Could you check a few things on this model? Use its own coordinates, in mm. A direction names the side the tool comes from. Give positions to 0.01 mm unless a question says otherwise; leave off trailing zeros. Order: outer loops, then holes, each group sorted by start corner. A loop starts at its lowest first (then second) coordinate and runs counter-clockwise, first axis right, second up.
from build123d import *

# Parameters (mm, degrees)
ENL_V_MAT_EXTRU_1_DEPTH = 0.5
CONG_1_R                = 0.2
CONG_2_R                = 1


# Read off the part's stored shape, not the designer's step: M5 Filetages mécaniques Borne1
with BuildPart() as part:
    # Esquisse1 → Révolution1 (revolve)
    with BuildSketch(Plane.XY):
        with BuildLine():
            Line((0, 0), (-7, 0))
            ThreePointArc((-7, 0), (-6.746211251, 2.061552813), (-6, 4))
            Line((-6, 4), (-5, 4))
            Line((-5, 4), (-5, 3))
            Line((-5, 3), (0, 3))
            Line((0, 3), (0, 0))
        make_face()
    revolve(axis=Axis((0, 0, 0), (-1, 0, 0)))

    # Esquisse2 → Enlèv. mat.-Extru.1 (cut)
    with BuildSketch(Plane.ZY.offset(7)):
        Polygon((0.75, 1.299038106), (-0.75, 1.299038106), (-1.5, 0), (-0.75, -1.299038106), (0.75, -1.299038106), (1.5, 0), align=None)
    extrude(amount=-ENL_V_MAT_EXTRU_1_DEPTH, mode=Mode.SUBTRACT)

    # Congé1
    cong_1_edges = [part.edges().sort_by_distance(p)[0] for p in [
        (-5, -3, 0),
    ]]
    fillet(cong_1_edges, radius=CONG_1_R)

    # Congé2
    cong_2_edges = [part.edges().sort_by_distance(p)[0] for p in [
        (-6, -4, 0),
    ]]
    fillet(cong_2_edges, radius=CONG_2_R)

    # M5 Filetages mécaniques Borne1 outline → M5 Filetages mécaniques Borne1 (revolve, cut)
    with BuildSketch(Plane.YX):
        Polygon((3, 0), (2.055, 0), (2.5, -0.445), (2.5, -4.8), (3, -4.8), align=None)
    revolve(axis=Axis((0, 0, 0), (1, 0, 0)), mode=Mode.SUBTRACT)


solid = part.part
Item 1: For pin 1 (3 mm diameter, centred on y = -1.5, z = 0, fed in from +X); pin 2 (4 mm diameter, centred on x = -1, y = -2, fed in from -Z); pin 3 (1.5 mm diameter, centred on x = -5, z = -1, fed in from -Y), each with a flat end and sliding along its axis, tell me the tip position at first contact or that it passes through.
Findings:
pin 1: stops at x = 0
pin 2: stops at z = -2.5
pin 3: stops at y = -3.99
Item 2: For faces 1 (the flat face through (-4.8, 2, 2)), 2 (the flat face through (0, 0, 0)), which set-ups out of +Z, -Z, +X, -X, +Y, -Y let a thin tool reach every point of the face, with its end or its side?
Findings:
face 1: +X
face 2: +Z, -Z, +X, +Y, -Y
Item 3: We'd pull the mould along Y, two halves only. Please class faces 3 (the cylindrical face through (-2.65, -0.54, -2.44)), 4 (the flat face through (-6.5, 0, 0)), 5 (the flat face through (-5, -2, -3)): +Y half, -Y half, draft (parallel to the pull), parting line (faces both ways), or undercut.
Findings:
face 3: parting line
face 4: undercut
face 5: draft
Item 4: Please list where these lines run through material, in increasing order: line 1 along Y through (x, z) = (-2.5, -2); line 2 along X through (y, z) = (-2, 2.75); line 3 along X through (y, z) = (0.75, -2.25).
Findings:
line 1: y = -1.5 to 1.5
line 2: x = -6.29 to -5
line 3: x = -6.66 to -0.32
Item 5: Imagine slicing it at A-A on x = -2. List the corners of the cut face in (y, z) for me.
Findings:
outline: circle Ø5 at (0, 0)
